from build123d import *

# Parameters (mm, degrees)
SKETCH_R      = 4.75
PAD_DEPTH     = 5
FILLET_R      = 10
FILLET001_R   = 1
SKETCH001_R   = 2
SKETCH001_W   = 9.475223
SKETCH001_H   = 23.68809
SKETCH001_W_2 = 11
SKETCH001_W_3 = 4.903309
SKETCH001_H_2 = 2.2
POCKET_DEPTH  = 5
SKETCH002_W   = 8
SKETCH002_H   = 4
PAD001_DEPTH  = 5
FILLET002_R   = 1.5


with BuildPart() as part:
    # Sketch → Pad (new body)
    with BuildSketch(Plane.XY):
        Polygon((30.887989, 10.25), (30.887989, 16.25), (-39.112011, 16.25), (-39.112011, -16.25), (30.887989, -16.25), (30.887989, -10.25), (10.887989, -10.25), (10.887989, 10.25), align=None)
        with Locations((-16.112011, 0)):
            Circle(SKETCH_R, mode=Mode.SUBTRACT)
    extrude(amount=PAD_DEPTH)

    # Fillet
    fillet_edges = [part.edges().sort_by_distance(p)[0] for p in [
        (-39.112011, -16.25, 2.5),
        (-39.112011, 16.25, 2.5),
    ]]
    fillet(fillet_edges, radius=FILLET_R)

    # Fillet001
    fillet001_edges = [part.edges().sort_by_distance(p)[0] for p in [
        (30.887989, -16.25, 2.5),
        (30.887989, 16.25, 2.5),
    ]]
    fillet(fillet001_edges, radius=FILLET001_R)

    # Sketch001 (on Face5 of Fillet001) → Pocket (cut)
    with BuildSketch(Plane.XY.offset(5)):
        with Locations((6.887989, 6.25)):
            Circle(SKETCH001_R)
        with Locations((6.887989, -6.25)):
            Circle(SKETCH001_R)
        with Locations((-28.9485835, 0)):
            Rectangle(SKETCH001_W, SKETCH001_H)
        with Locations((-2.4204911845, 0)):
            Rectangle(SKETCH001_W_2, SKETCH001_H)
        with Locations((8.4363345, 0)):
            Rectangle(SKETCH001_W_3, SKETCH001_H_2)
    extrude(amount=-POCKET_DEPTH, mode=Mode.SUBTRACT)

    # Sketch002 (on Face5 of Pocket) → Pad001 (join)
    with BuildSketch(Plane.XY.offset(5)):
        with Locations((-16.112011, 9.067142847)):
            Rectangle(SKETCH002_W, SKETCH002_H)
        with Locations((-16.112011, -9.067142847)):
            Rectangle(SKETCH002_W, SKETCH002_H)
    extrude(amount=PAD001_DEPTH)

    # Fillet002
    fillet002_edges = [part.edges().sort_by_distance(p)[0] for p in [
        (-16.112011, 11.067143, 10),
        (-12.112011, 9.067143, 10),
        (-16.112011, 7.067143, 10),
        (-20.112011, 9.067143, 10),
        (-16.112011, -7.067143, 10),
        (-12.112011, -9.067143, 10),
        (-16.112011, -11.067143, 10),
        (-20.112011, -9.067143, 10),
    ]]
    fillet(fillet002_edges, radius=FILLET002_R)


solid = part.part
Work out the finished part from the listing and answer in its coordinate system (mm). A direction names the side the tool comes from. Round coordinates to 2 decimals unless told otherwise and drop trailing zeros. Write each loop counter-clockwise with the first axis right and the second up, starting at its lowest first coordinate (ties: lowest second). Pieces come first, ordered by that corner, then holes. Notation, with made-up numbers: (-22.5, -27) - (0.5, -27) arc R12 cw to (0.5, -4) - close; hole circle Ø3 at (-12, -6.75). An arc over 180 degrees is marked (long way). Answer in a Markdown table with one row per item. Add a question column.
1. A cutting plane is placed at A-A, the plane x = -1. Determine the outline of the cut face in (y, z).
2. A cutting plane is placed at B-B, the plane y = 0. Determine the outline of the cut face in (x, z).
3. A cutting plane is placed at D-D, the plane z = 7.25. Determine the outline of the cut face in (x, y), and give its area (3 significant figures).
4. Find the intervals of material crossed by line 1 along Y through (x, z) = (18.5, 3.5); line 2 along X through (y, z) = (-6.5, 3); line 3 along Y through (x, z) = (9, 0.75), in increasing order. Write a range as from..to.
5. For faces 4 (the flat face through (-16, 11.067, 7)), 5 (the flat face through (8, 1.1, 3)), 6 (the flat face through (-12.112, 9, 7)), 7 (the flat face through (-16, -7.067, 7)), 8 (the flat face through (-20.112, 9, 7)), determine the directions among +Z, -Z, +X, -X, +Y, -Y from which every point of the face is accessible in a straight line to the end or side of a thin tool.
6. The mould has two halves that part along X. Classify faces 1 (the flat face through (30.888, 13, 2)), 2 (the cylindrical face through (8.796, 6.851, 2.535)), 3 (the cylindrical face through (-36.105, 13.398, 2.535)): +X half, -X half, draft (parallel to the pull), parting line (faces both ways), or undercut.
7. A cutting plane is placed at C-C, the plane z = 1. Determine the outline of the cut face in (x, y), and give its area (3 significant figures).
8. Given pin 1 (1.8 mm diameter, centred on y = 9, z = 6.5, fed in from +X); pin 2 (12.5 mm diameter, centred on x = -16.11, y = 0, fed in from +Z); pin 3 (1.8 mm diameter, centred on y = -8, z = 7.5, fed in from -X); pin 4 (6 mm diameter, centred on y = 7.5, z = 5.5, fed in from -X), each flat-ended and moving along its own axis, determine where each tip first touches the part or whether it passes through.
Worked out:
| question | item | result |
|---|---|---|
| 1 | outline | (-16.25, 0) - (-11.84, 0) - (-11.84, 5) - (-16.25, 5) - close; (11.84, 0) - (16.25, 0) - (16.25, 5) - (11.84, 5) - close |
| 2 | outline | (-39.11, 0) - (-33.69, 0) - (-33.69, 5) - (-39.11, 5) - close; (-24.21, 0) - (-20.86, 0) - (-20.86, 5) - (-24.21, 5) - close; (-11.36, 0) - (-7.92, 0) - (-7.92, 5) - (-11.36, 5) - close; (3.08, 0) - (5.98, 0) - (5.98, 5) - (3.08, 5) - close |
| 3 | outline | (-20.11, -11.07) - (-12.11, -11.07) - (-12.11, -7.07) - (-20.11, -7.07) - close; (-20.11, 7.07) - (-12.11, 7.07) - (-12.11, 11.07) - (-20.11, 11.07) - close |
| 3 | area | 64.0 mm^2 |
| 4 | line 1 | -16.25..-10.25, 10.25..16.25 |
| 4 | line 2 | -39.11..-33.69, -24.21..-7.92, 3.08..4.9, 8.87..10.89 |
| 4 | line 3 | -16.25..-1.1, 1.1..16.25 |
| 5 | face 4 | +Z, +X, -X, +Y |
| 5 | face 5 | +Z, -Z, +X |
| 5 | face 6 | +Z, +X, +Y, -Y |
| 5 | face 7 | +Z, +X, -X |
| 5 | face 8 | +Z, -X, +Y, -Y |
| 6 | face 1 | +X half |
| 6 | face 2 | undercut |
| 6 | face 3 | -X half |
| 7 | outline | (-39.11, -6.25) arc R10 ccw to (-29.11, -16.25) - (29.89, -16.25) arc R1 ccw to (30.89, -15.25) - (30.89, -10.25) - (10.89, -10.25) - (10.89, -1.1) - (5.98, -1.1) - (5.98, 1.1) - (10.89, 1.1) - (10.89, 10.25) - (30.89, 10.25) - (30.89, 15.25) arc R1 ccw to (29.89, 16.25) - (-29.11, 16.25) arc R10 ccw to (-39.11, 6.25) - close; hole (-33.69, -11.84) - (-24.21, -11.84) - (-24.21, 11.84) - (-33.69, 11.84) - close; hole circle Ø9.5 at (-16.11, 0); hole (-7.92, -11.84) - (3.08, -11.84) - (3.08, 11.84) - (-7.92, 11.84) - close; hole circle Ø4 at (6.89, -6.25); hole circle Ø4 at (6.89, 6.25) |
| 7 | area | 1,230 mm^2 |
| 8 | pin 1 | x = -12.11 |
| 8 | pin 2 | z = 5 |
| 8 | pin 3 | x = -20.11 |
| 8 | pin 4 | x = -39.11 |
